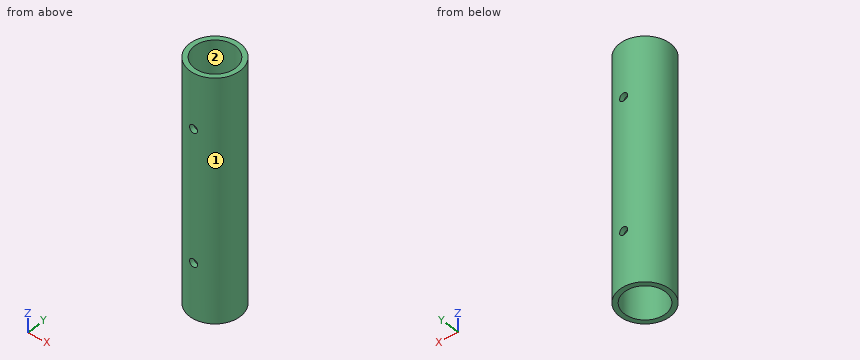
Autodesk Inventor part; units mm, degrees
ref_plane "Work Plane4" through (0, 18.5, 0) normal (0, 1, 0) x (-1, 0, 0)
ref_plane "YZ Plane" through (0, 0, 0) normal (1, 0, 0) x (0, 1, 0)
ref_plane "XZ Plane" through (0, 0, 0) normal (0, 1, 0) x (-1, 0, 0)
sketch "Sketch1" plane through (0, 0, 0) normal (0, 0, 1) x (1, 0, 0)
  circle A0 centre (0, 0) radius 18.5
  circle A1 centre (0, 0) radius 15
  dimension "d0" = 37
  dimension "d1" = 30
extrude "Extrusion1" add sketch "Sketch1" along normal mid plane 178
ref_plane "Work Plane4" through (0, 18.5, 0) normal (0, 1, 0) x (-1, 0, 0)
sketch "Sketch4" plane through (0, 18.5, 0) normal (0, 1, 0) x (-1, 0, 0)
  line L0 (-18.5, -89) -> (18.5, -89)
  line L1 (18.5, -89) -> (18.5, 89)
  line L2 (-18.5, -89) -> (18.5, -89)
  line L3 (18.5, 89) -> (-18.5, 89)
  point P0 (0, 0)
  point P1 (0, -48.5)
  dimension "d14" = 40.5
  dimension "d22" = 178
  dimension "d23" = 18.5
hole "Hole1" at (0, 18.5, -48.5) direction (0, -1, 0) diameter 5.9175 depth 19.1 tip angle 118
mirror "Mirror1" about plane through (0, 0, 0) normal (0, 0, 1) of "Hole1"
mirror "Mirror2" about plane through (0, 0, 0) normal (0, 1, 0) of "Hole1", "Mirror1"
properties part number "EjeRodilla"
Verification items for the finished model (mm, model axes). Face numbers are marked on the shaded views. Coordinates: 2 decimals unless noted, no trailing zeros. Order: outer loops, then holes, each group sorted by start corner. A loop starts at its lowest first (then second) coordinate and runs counter-clockwise, first axis right, second up. Notation, with made-up numbers: M -6,-7 L 16,-7 A16 ccw 16,-3 Z; hole C -20.75,6.25 d10. An arc over 180 degrees is marked long. Write each question's results on one line, items separated by ' | '.
1) Scan lines: line 1 along Z through (x, y) = (0, -15.55); line 2 along Y through (x, z) = (0.5, -82); line 3 along Y through (x, z) = (13.5, -52). Record each from-to range of solid material in increasing order. Write a range as [from, to].
Solved:
line 1: z = [-89, -51.46], [-45.54, 45.54], [51.46, 89] | line 2: y = [-18.49, -14.99], [14.99, 18.49] | line 3: y = [-12.65, -6.54], [6.54, 12.65]
2) Section check C-C on z = -23.5. Record the cut outline in (x, y).
Solved:
outline: C 0,0 d37; hole C 0,0 d30
3) Release check for a two-part mould opening along Y. For the marked faces 1 and 2 record: pulls with the +Y half, pulls with the -Y half, needs draft (parallel to the pull), parting line crosses it, or undercut.
Solved:
face 1: parting line crosses it | face 2: undercut
4) Section check D-D on x = -10. Record the cut outline in (y, z), plus the area to 3 significant figures.
Solved:
outline: M -15.56,-89 L -11.18,-89 L -11.18,89 L -15.56,89 Z; M 11.18,-89 L 15.56,-89 L 15.56,89 L 11.18,89 Z | area: 1,560 mm²
5) Section check A-A on y = 0. Record the cut outline in (x, z), plus the area to 3 significant figures.
Solved:
outline: M -18.5,-89 L -15,-89 L -15,89 L -18.5,89 Z; M 15,-89 L 18.5,-89 L 18.5,89 L 15,89 Z | area: 1,250 mm²
6) Gauge pin test, flat ends, axial feed: pin 1 Ø12 at (x, z) = (7.5, -41) entering from +Y; pin 2 Ø3 at (y, z) = (-3.5, -55) entering from +X; pin 3 Ø1 at (y, z) = (-11.5, 21) entering from +X. Record the tip position at first contact, or that the pin passes through.
Solved:
pin 1: stops at y = 18.44 | pin 2: stops at x = 18.39 | pin 3: stops at x = 14.87
7) Section check B-B on x = 0. Record the cut outline in (y, z), plus the area to 3 significant figures.
Solved:
outline: M -18.5,-89 L -15,-89 L -15,-51.46 L -18.5,-51.46 Z; M -18.5,-45.54 L -15,-45.54 L -15,45.54 L -18.5,45.54 Z; M -18.5,51.46 L -15,51.46 L -15,89 L -18.5,89 Z; M 15,-89 L 18.5,-89 L 18.5,-51.46 L 15,-51.46 Z; M 15,-45.54 L 18.5,-45.54 L 18.5,45.54 L 15,45.54 Z; M 15,51.46 L 18.5,51.46 L 18.5,89 L 15,89 Z | area: 1,160 mm²
